```python
from build123d import *

# Parameters (mm, degrees)
F0_R     = 4.2
F1_DEPTH = 0.85
F3_DEPTH = 2.55
F4_R     = 1.69999
F5_R     = 0.85
F6_DEPTH = 25


# Not quite as in the source:
# - a fillet or chamfer is up to 0.001 mm smaller than in the source, because OpenCascade refuses the exact size


with BuildPart() as f1:
    # F0 (on Top) → F1 (new body)
    with BuildSketch(Plane.XY):
        with BuildLine():
            Line((16.0373335058, 4.3), (20.2, 4.3))
            Line((20.2, 4.3), (20.2, 7.7))
            Line((20.2, 7.7), (16.0373335058, 7.7))
            ThreePointArc((16.0373335058, 7.7), (14.2805243712, 7.9629605488), (12.6777057346, 8.7287927785))
            Line((12.6777057346, 8.7287927785), (9.3596277711, 10.9712072215))
            ThreePointArc((9.3596277711, 10.9712072215), (7.7568091346, 11.7370394512), (6, 12))
            ThreePointArc((6, 12), (1.7573593129, 10.2426406871), (0, 6))
            ThreePointArc((0, 6), (1.7573593129, 1.7573593129), (6, 0))
            ThreePointArc((6, 0), (7.7568091346, 0.2629605488), (9.3596277711, 1.0287927785))
            Line((9.3596277711, 1.0287927785), (12.6777057346, 3.2712072215))
            ThreePointArc((12.6777057346, 3.2712072215), (14.2805243712, 4.0370394512), (16.0373335058, 4.3))
        make_face()
        with Locations((6, 6)):
            Circle(F0_R, mode=Mode.SUBTRACT)
    extrude(amount=F1_DEPTH)

    # F2 (on face) → F3 (join)
    with BuildSketch(Plane.XY.offset(0.85)):
        Polygon((20.2, 4.3), (20.2, 7.7), (16.0373335058, 7.7), (15.7, 7.7), (15.7, 4.3), (16.0373335058, 4.3), align=None)
    extrude(amount=F3_DEPTH)

    # F4 (radius 1.7 in the source; OpenCascade refuses exactly that, so slightly less here)
    f4_edges = [f1.edges().sort_by_distance(p)[0] for p in [
        (17.95, 7.7, 3.4),
        (17.95, 4.3, 3.4),
    ]]
    fillet(f4_edges, radius=F4_R)

    # F5 (on face) → F6 (cut)
    with BuildSketch(Plane.YZ.offset(20.2)):
        with Locations((6, 1.7)):
            Circle(F5_R)
    extrude(amount=-F6_DEPTH, mode=Mode.SUBTRACT)


solid = f1.part
```
Could you check a few things on this model? Use its own coordinates, in mm. A direction names the side the tool comes from. Round coordinates to 2 decimals unless told otherwise and drop trailing zeros. Loops run counter-clockwise (first coordinate to the right, second up) from the corner with the lowest first, then second, coordinate; pieces in that order, holes last. Notation, with made-up numbers: M 46.5,27 L 77.5,27 A33 ccw 77.5,60 Z; hole C 37.5,-3 d10. An arc over 180 degrees is marked long. Write item = value, one per line.
1. I want a section at A-A, the plane x = 6.75. Write out the boundary of the cut face in (y, z), and give its area (3 significant figures).
Results below:
outline = M 0.05,0 L 1.87,0 L 1.87,0.85 L 0.05,0.85 Z; M 10.13,0 L 11.95,0 L 11.95,0.85 L 10.13,0.85 Z
area = 3.09 mm²
2. Which directions (+Z, -Z, +X, -X, +Y, -Y) give clear straight access to the entire face, cutting with the end or side of a thin tool? Please do faces 5 (the face through (18, 7.7, 1)), 6 (the face through (15.7, 6, 3)), 7 (the face through (14.26, 4.03, 0.42)).
Results below:
face_5 = +Z, -Z, +X, +Y
face_6 = +Z, -X, +Y, -Y
face_7 = +Z, -Z, +X, -Y
3. I want a section at C-C, the plane z = 0.45. Write out the boundary of the cut face in (x, y), and give its area (3 significant figures).
Results below:
outline = M 9.36,1.03 L 12.68,3.27 A6 cw 16.04,4.3 L 20.2,4.3 L 20.2,7.7 L 16.04,7.7 A6 cw 12.68,8.73 L 9.36,10.97 A6 ccw long Z; hole C 6,6 d8.4
area = 92.6 mm²
4. I need wall thicknesses on probe 1 along Y at (x, z) = (6, 0.6); probe 2 along X at (y, z) = (6, 0.4); probe 3 along Z at (x, y) = (18.55, 6). Which ranges of each line are inside material? Lowest first, please.
Results below:
probe_1 = 0 to 1.8, 10.2 to 12
probe_2 = 0 to 1.8, 10.2 to 20.2
probe_3 = 0 to 0.85, 2.55 to 3.4
5. Thinking about a two-plate mould opening in Y: for faces 1 (the face through (10, 9, 0.85)), 2 (the face through (18, 4.3, 1)), 3 (the face through (7.938, 2.274, 0.419)), 4 (the face through (14.304, 7.956, 0.419)), which applies, +Y half, -Y half, draft (parallel to the pull), parting line (faces both ways), or undercut?
Results below:
face_1 = draft
face_2 = -Y half
face_3 = undercut
face_4 = +Y half
6. Will these pins go through, and if not, where does the flat tip stop? P1, Ø0.9, axis at x = 18.5, z = 0.5, coming from the +Y side; P2, Ø1.9, axis at x = 17, z = 1, coming from the -Y side; P3, Ø1, axis at y = 3, z = 1, coming from the -X side.
Results below:
P1 = 7.7
P2 = 4.3
P3 = 0.56
7. I want a section at B-B, the plane y = 6.5. Write out the boundary of the cut face in (x, z), and give its area (3 significant figures).
Results below:
outline = M 0.02,0 L 1.83,0 L 1.83,0.85 L 0.02,0.85 Z; M 10.17,0 L 20.2,0 L 20.2,1.01 L 15.7,1.01 L 15.7,0.85 L 10.17,0.85 Z; M 15.7,2.39 L 20.2,2.39 L 20.2,3.32 L 15.7,3.32 Z
area = 15.0 mm²
8. I want a section at D-D, the plane y = 4.75. Write out the boundary of the cut face in (x, z), and give its area (3 significant figures).
Results below:
outline = M 0.13,0 L 1.99,0 L 1.99,0.85 L 0.13,0.85 Z; M 10.01,0 L 20.2,0 L 20.2,2.85 L 15.7,2.85 L 15.7,0.85 L 10.01,0.85 Z
area = 19.3 mm²
